CAD build for the part. Positions are in the model's coordinates, mm. A direction names the side the tool comes from. Coordinates: 2 decimals unless noted, no trailing zeros. Order: outer loops, then holes, each group sorted by start corner. A loop starts at its lowest first (then second) coordinate and runs counter-clockwise, first axis right, second up. Notation, with made-up numbers: (74, -38.75) - (89, -38.75) arc R14 ccw to (89, -18.75) - close; hole circle Ø10 at (17.25, 31). An arc over 180 degrees is marked (long way). Return JSON: item names as keys, results as strings.
Autodesk Inventor part; units mm, degrees
ref_plane "YZ Plane" through (0, 0, 0) normal (1, 0, 0) x (0, 1, 0)
ref_plane "XZ Plane" through (0, 0, 0) normal (0, 1, 0) x (-1, 0, 0)
ref_plane "XY Plane" through (0, 0, 0) normal (0, 0, 1) x (1, 0, 0)
sketch "Sketch1" plane through (0, 0, 0) normal (0, 0, 1) x (1, 0, 0)
  arc A0 (0, 3) -> (3, 0) centre (3.0011, 3.0011) ccw
  line L0 (3, 0) -> (15.44, 0)
  arc A1 (22.577, -1.806) -> (15.44, 0) centre (15.444, -14.9894) ccw
  line L1 (22.577, -1.806) -> (29.869, -5.751)
  arc A2 (29.869, -5.751) -> (55.947, -0.778) centre (39.8598, 12.7202) ccw
  line L2 (55.947, -0.778) -> (85.929, 34.955)
  arc A3 (115.145, 36.485) -> (85.929, 34.955) centre (101.2502, 22.1018) ccw
  line L3 (115.145, 36.485) -> (145.651, 7.018)
  arc A4 (145.651, 7.018) -> (163.02, 0) centre (163.0155, 24.9912) ccw
  line L4 (163.02, 0) -> (182, 0)
  arc A5 (182, 0) -> (185, 3) centre (181.9989, 3.0011) ccw
  line L5 (0, 3) -> (0, 21.1)
  arc A6 (3, 24.1) -> (0, 21.1) centre (3.0011, 21.0989) ccw
  line L6 (3, 24.1) -> (12.73, 24.1)
  arc A7 (24.609, 21.097) -> (12.73, 24.1) centre (12.7244, -0.9184) ccw
  line L7 (24.609, 21.097) -> (30.766, 17.772)
  arc A8 (30.766, 17.772) -> (55.59, 22.514) centre (40.2694, 35.3692) ccw
  line L8 (55.59, 22.514) -> (85.294, 57.909)
  arc A9 (115.968, 59.516) -> (85.294, 57.909) centre (101.3803, 44.4098) ccw
  line L9 (115.968, 59.516) -> (148.28, 28.31)
  arc A10 (148.28, 28.31) -> (158.7, 24.1) centre (158.6991, 39.0977) ccw
  line L10 (158.7, 24.1) -> (182, 24.1)
  arc A11 (185, 21.1) -> (182, 24.1) centre (181.9989, 21.0989) ccw
  line L11 (185, 21.1) -> (185, 3)
extrude "Extrusion1" add sketch "Sketch1" along normal mid plane 1
properties part number "Offset"
Item 1: Band-saw the part on D-D, the plane x = 154. List the corners of the cut face in (y, z), then the cut area to 3 significant figures.
Findings below:
{"outline": "(1.68, -0.5) - (24.86, -0.5) - (24.86, 0.5) - (1.68, 0.5) - close", "area": "23.2 mm²"}
Item 2: Band-saw the part on A-A, the plane y = 11. List the corners of the cut face in (x, z), then the cut area to 3 significant figures.
Findings below:
{"outline": "(0, -0.5) - (65.83, -0.5) - (65.83, 0.5) - (0, 0.5) - close; (141.53, -0.5) - (185, -0.5) - (185, 0.5) - (141.53, 0.5) - close", "area": "109 mm²"}
Item 3: Which spindle directions (+Z, -Z, +X, -X, +Y, -Y) get a long thin tool onto all of the face, cutting with end or side? Do faces 4 (the flat face through (130.18, 21.96, -0.01)), 5 (the cylindrical face through (184.1, 23.24, -0.01)), 6 (the flat face through (27.64, 19.46, -0.01)). Say none if no direction does.
Findings below:
{"face 4": "+Z, -Z, -Y", "face 5": "+Z, -Z, +X, +Y", "face 6": "+Z, -Z, +Y"}
Item 4: Mould opens along X. For faces 1 (the cylindrical face through (43.99, -7.87, -0.01)), 2 (the cylindrical face through (18.77, 23.36, -0.01)), 3 (the cylindrical face through (0.9, 0.86, -0.01)) say: released by +X, released by -X, zero draft, split by the parting line, or undercut.
Findings below:
{"face 1": "split by the parting line", "face 2": "undercut", "face 3": "released by -X"}
Item 5: Wall check: L1, parallel to Y at x = 12.5, z = -0.3; L2, parallel to X at y = 27.5, z = -0.3; L3, parallel to X at y = 21.5, z = -0.05. Give the ranges that are in metal, low to high. Write a range as [from, to].
Findings below:
{"L1": "y = [0, 24.1]", "L2": "x = [59.77, 79.67], [124.45, 149.19]", "L3": "x = [0.03, 23.83], [54.68, 74.64], [130.66, 184.97]"}
Item 6: Band-saw the part on C-C, the plane x = 113.5. List the corners of the cut face in (y, z), then the cut area to 4 significant figures.
Findings below:
{"outline": "(37.91, -0.5) - (61.56, -0.5) - (61.56, 0.5) - (37.91, 0.5) - close", "area": "23.65 mm²"}
Item 7: Band-saw the part on B-B, the plane z = 0.3. List the corners of the cut face in (x, y) (3 decimals).
Findings below:
{"outline": "(0, 3) arc R3.001 ccw to (3, 0) - (15.44, 0) arc R14.99 cw to (22.577, -1.806) - (29.869, -5.751) arc R21 ccw to (55.947, -0.778) - (85.929, 34.955) arc R19.999 cw to (115.145, 36.485) - (145.651, 7.018) arc R24.991 ccw to (163.02, 0) - (182, 0) arc R3.001 ccw to (185, 3) - (185, 21.1) arc R3.001 ccw to (182, 24.1) - (158.7, 24.1) arc R14.997 cw to (148.28, 28.31) - (115.968, 59.516) arc R21 ccw to (85.294, 57.909) - (55.59, 22.514) arc R19.999 cw to (30.766, 17.772) - (24.609, 21.097) arc R25.018 ccw to (12.73, 24.1) - (3, 24.1) arc R3.001 ccw to (0, 21.1) - close"}
